```python
from build123d import *

# Parameters (mm, degrees)
BOSS_EXTRU_1_DEPTH      = 8.5598
ESQUISSE2_R             = 4.7625
ENL_V_MAT_EXTRU_1_DEPTH = 14.86894224


with BuildPart() as part:
    # Esquisse1 → Boss.-Extru.1 (new body)
    with BuildSketch(Plane(origin=(0, 0, 0), x_dir=(1, 0, 0), z_dir=(0, 1, 0))):
        Polygon((4.124445986, 7.14375), (-4.124445986, 7.14375), (-8.248891971, 0), (-4.124445986, -7.14375), (4.124445986, -7.14375), (8.248891971, 0), align=None)
    extrude(amount=BOSS_EXTRU_1_DEPTH)

    # Esquisse2 → Enlèv. mat.-Extru.1 (cut, through all)
    with BuildSketch(Plane(origin=(0, 8.5598, 0), x_dir=(1, 0, 0), z_dir=(0, 1, 0))):
        with Locations(Location((0, 0, 0), (0, 0, 270))):
            Circle(ESQUISSE2_R)
    extrude(amount=-ENL_V_MAT_EXTRU_1_DEPTH, mode=Mode.SUBTRACT)

    # Esquisse6 → Enlèvement de matière-Révolution1 (revolve, cut)
    with BuildSketch(Plane.XY, mode=Mode.PRIVATE) as enl_vement_de_mati_re_r_volution1_sk:
        with BuildLine():
            Line((-8.248891971, 8.5598), (-7.086761314, 8.5598))
            Line((-7.086761314, 8.5598), (-5.924630657, 8.5598))
            ThreePointArc((-5.924630657, 8.5598), (-7.427141503, 7.738049532), (-8.248891971, 6.235538686))
            Line((-8.248891971, 6.235538686), (-8.248891971, 7.397669343))
            Line((-8.248891971, 7.397669343), (-8.248891971, 8.5598))
        make_face()
    revolve(enl_vement_de_mati_re_r_volution1_sk.sketch.rotate(Axis((0, 0, 0), (0, 1, 0)), 270), axis=Axis((0, 0, 0), (0, 1, 0)), mode=Mode.SUBTRACT)


solid = part.part
```
The model under review builds one solid part; all positions refer to its coordinate system, in mm. Round coordinates to 2 decimals unless told otherwise and drop trailing zeros. Order: outer loops, then holes, each group sorted by start corner. A loop starts at its lowest first (then second) coordinate and runs counter-clockwise, first axis right, second up. Notation, with made-up numbers: M 39,62.25 L 56,62.25 A22 ccw 56,99.25 Z; hole C -30.5,17.5 d1. An arc over 180 degrees is marked long. Use a Markdown table: item, result.
1) Draft analysis for pull direction X (two halves, no side actions). For faces 1 (the face through (-2.9, 4.34, -3.78)), 2 (the face through (0, 4, 7.144)), 3 (the face through (-6.216, 3.938, 3.522)), 4 (the face through (6.16, 3.94, 3.62)), state which applies: released by +X, released by -X, zero draft, split by the parting line, or undercut.
Report:
| item | result |
|---|---|
| face 1 | undercut |
| face 2 | zero draft |
| face 3 | released by -X |
| face 4 | released by +X |
2) Insertion check: pin 1 (4 mm diameter, centred on y = 6, z = -3.5, fed in from -X); pin 2 (2 mm diameter, centred on x = -5, z = -5, fed in from -Y); pin 3 (1.5 mm diameter, centred on y = 2, z = -1.5, fed in from +X); pin 4 (4 mm diameter, centred on y = 6.5, z = -4.5, fed in from +X). Each pin has a flat end and moves straight along its axis. Give the tip position at first contact, or say it passes through.
Report:
| item | result |
|---|---|
| pin 1 | x = -7.38 |
| pin 2 | y = 0 |
| pin 3 | x = 7.82 |
| pin 4 | x = 6.81 |
3) Consider section A-A (y = 2). Write out the cut boundary in (x, z) (1 decimal).
Report:
| item | result |
|---|---|
| outline | M -8.2,0 L -4.1,-7.1 L 4.1,-7.1 L 8.2,0 L 4.1,7.1 L -4.1,7.1 Z; hole C 0,0 d9.5 |
4) Consider section B-B (x = 0). Write out the cut boundary in (y, z).
Report:
| item | result |
|---|---|
| outline | M 0,-7.14 L 7.99,-7.14 A3.05 ccw 8.56,-5.92 L 8.56,-4.76 L 0,-4.76 Z; M 0,4.76 L 8.56,4.76 L 8.56,5.92 A3.05 ccw 7.99,7.14 L 0,7.14 Z |
5) Consider section C-C (y = 7). Write out the cut boundary in (x, z) (1 decimal).
Report:
| item | result |
|---|---|
| outline | M -8,-0.5 L -4.4,-6.6 A8 ccw -3.5,-7.1 L 3.5,-7.1 A8 ccw 4.4,-6.6 L 8,-0.5 A8 ccw 8,0.5 L 4.4,6.6 A8 ccw 3.5,7.1 L -3.5,7.1 A8 ccw -4.4,6.6 L -8,0.5 A8 ccw Z; hole C 0,0 d9.5 |
6) Wall thickness on line 1 along X through (y, z) = (6.5, 0); line 2 along Z through (x, y) = (3.25, 2.75); line 3 along X through (y, z) = (1, 2.5): over which ranges is each line inside the solid? List them lowest first. Write a range as [from, to].
Report:
| item | result |
|---|---|
| line 1 | [-8.18, -4.76], [4.76, 8.18] |
| line 2 | [-7.14, -3.48], [3.48, 7.14] |
| line 3 | [-6.81, -4.05], [4.05, 6.81] |
